Can you work these out from the model? Positions are in its coordinate system, mm. Face numbers are marked on the shaded views. Give positions to 0.01 mm unless a question says otherwise; leave off trailing zeros. Order: outer loops, then holes, each group sorted by start corner. A loop starts at its lowest first (then second) coordinate and runs counter-clockwise, first axis right, second up. Notation, with made-up numbers: (8.5, -38.5) - (61.5, -38.5) arc R22 cw to (61.5, -26.5) - close; hole circle Ø5 at (7.5, -24.5). An arc over 180 degrees is marked (long way). One line per question, with ' | ' between items.
```python
from build123d import *

# Parameters (mm, degrees)
F0_W     = 75
F0_H     = 65
F0_R     = 22.5
F1_DEPTH = 32.5
F2_R     = 4
F3_DEPTH = 65.001
F2_R_2   = 7
F4_DEPTH = 5


with BuildPart() as f1:
    # F0 (on Front) → F1 (new body, symmetric)
    with BuildSketch(Plane.XZ):
        with Locations((37.5, 32.5)):
            Rectangle(F0_W, F0_H)
        with Locations((37.5, 32.5)):
            Circle(F0_R, mode=Mode.SUBTRACT)
    extrude(amount=F1_DEPTH, both=True)

    # F2 (on face) → F3 (cut, through all)
    with BuildSketch(Plane.XY.offset(65)):
        with Locations((66.5, 17.5)):
            Circle(F2_R)
        with Locations((66.5, -17.5)):
            Circle(F2_R)
        with Locations((8.5, -17.5)):
            Circle(F2_R)
        with Locations((8.5, 17.5)):
            Circle(F2_R)
    extrude(amount=-F3_DEPTH, mode=Mode.SUBTRACT)

    # F2 (on face) → F4 (cut)
    with BuildSketch(Plane.XY.offset(65)):
        with Locations((8.5, 17.5)):
            Circle(F2_R_2)
        with Locations((8.5, 17.5)):
            Circle(F2_R, mode=Mode.SUBTRACT)
        with Locations((66.5, 17.5)):
            Circle(F2_R_2)
        with Locations((66.5, 17.5)):
            Circle(F2_R, mode=Mode.SUBTRACT)
        with Locations((66.5, -17.5)):
            Circle(F2_R_2)
        with Locations((66.5, -17.5)):
            Circle(F2_R, mode=Mode.SUBTRACT)
        with Locations((8.5, -17.5)):
            Circle(F2_R_2)
        with Locations((8.5, -17.5)):
            Circle(F2_R, mode=Mode.SUBTRACT)
    extrude(amount=-F4_DEPTH, mode=Mode.SUBTRACT)


solid = f1.part
```
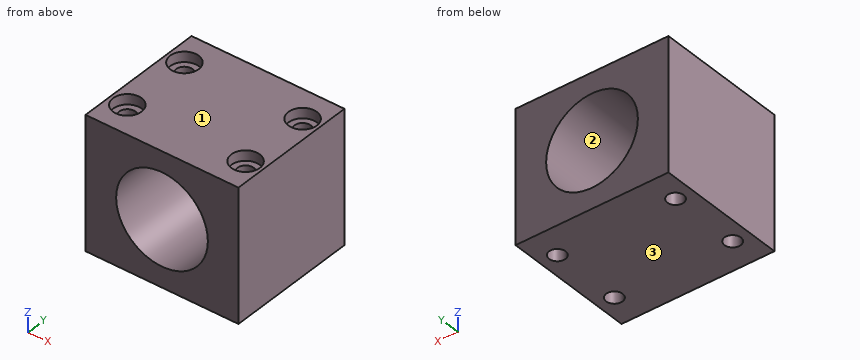
(1) If I drill on line 1 (X direction, y = -17, z = 61); line 2 (Y direction, x = 66, z = 62); line 3 (Y direction, x = 8.5, z = 37), over which ranges is the centre line in solid material (lowest first)?
Answer below:
line 1: 0 to 1.52, 15.48 to 59.52, 73.48 to 75 | line 2: -32.5 to -24.48, -10.52 to 10.52, 24.48 to 32.5 | line 3: -32.5 to -21.5, -13.5 to 13.5, 21.5 to 32.5
(2) Imagine slicing it at B-B (z = 32.5). List the corners of the cut face in (x, y) for me, and give its area (3 significant figures).
Answer below:
outline: (0, -32.5) - (15, -32.5) - (15, 32.5) - (0, 32.5) - close; (60, -32.5) - (75, -32.5) - (75, 32.5) - (60, 32.5) - close; hole circle Ø8 at (8.5, -17.5); hole circle Ø8 at (8.5, 17.5); hole circle Ø8 at (66.5, -17.5); hole circle Ø8 at (66.5, 17.5) | area: 1,750 mm^2
(3) If we mould it in two halves opening along Z, with no side actions, what happens to the marked faces 1, 2 and 3? For each: released by +Z, released by -Z, zero draft, split by the parting line, or undercut.
Answer below:
face 1: released by +Z | face 2: undercut | face 3: released by -Z
(4) Imagine slicing it at A-A (y = -17.5). List the corners of the cut face in (x, z) for me.
Answer below:
outline: (0, 0) - (4.5, 0) - (4.5, 60) - (1.5, 60) - (1.5, 65) - (0, 65) - close; (12.5, 0) - (62.5, 0) - (62.5, 60) - (59.5, 60) - (59.5, 65) - (15.5, 65) - (15.5, 60) - (12.5, 60) - close; (70.5, 0) - (75, 0) - (75, 65) - (73.5, 65) - (73.5, 60) - (70.5, 60) - close; hole circle Ø45 at (37.5, 32.5)
(5) Imagine slicing it at D-D (x = 8.5). List the corners of the cut face in (y, z) for me, and give its area (4 significant figures).
Answer below:
outline: (-32.5, 0) - (-21.5, 0) - (-21.5, 60) - (-24.5, 60) - (-24.5, 65) - (-32.5, 65) - close; (-13.5, 0) - (13.5, 0) - (13.5, 60) - (10.5, 60) - (10.5, 65) - (-10.5, 65) - (-10.5, 60) - (-13.5, 60) - close; (21.5, 0) - (32.5, 0) - (32.5, 65) - (24.5, 65) - (24.5, 60) - (21.5, 60) - close | area: 3,125 mm^2
(6) Will these pins go through, and if not, where does the flat tip stop? pin 1 (7 mm diameter, centred on x = 65.5, y = -18.5, fed in from +Z); pin 2 (6.5 mm diameter, centred on x = 8.5, y = -17.5, fed in from +Z).
Answer below:
pin 1: z = 60 | pin 2: through
(7) Imagine slicing it at C-C (z = 56.5). List the corners of the cut face in (x, y) for me, and give its area (3 significant figures).
Answer below:
outline: (0, -32.5) - (75, -32.5) - (75, 32.5) - (0, 32.5) - close; hole circle Ø8 at (8.5, -17.5); hole circle Ø8 at (8.5, 17.5); hole circle Ø8 at (66.5, -17.5); hole circle Ø8 at (66.5, 17.5) | area: 4,670 mm^2
